```python
from build123d import *

# Parameters (mm, degrees)
F0_W      = 6
F0_H      = 10
F1_DEPTH  = 2
F2_W      = 2.8
F2_H      = 10
F3_DEPTH  = 10
F4_DEPTH  = 3
F5_DEPTH  = 0.8
F7_DEPTH  = 25
F8_SIZE   = 0.5
F10_DEPTH = 63
F11_W     = 6
F11_H     = 2
F12_DEPTH = 10
F13_W     = 2.8
F13_H     = 10
F14_DEPTH = 10
F15_R     = 2.5
F16_DEPTH = 25
F17_SIZE  = 4
F18_W     = 2.8
F18_H     = 51
F19_DEPTH = 1


with BuildPart() as f1:
    # F0 (on Top) → F1 (new body)
    with BuildSketch(Plane.XY):
        with Locations((3, -5)):
            Rectangle(F0_W, F0_H)
    extrude(amount=F1_DEPTH)

    # F2 (on face) → F3 (join)
    with BuildSketch(Plane.XY.offset(2)):
        with Locations((3, -5)):
            Rectangle(F2_W, F2_H)
    extrude(amount=F3_DEPTH)

    # F4 (cut): a face of the model
    f4_faces = [f1.faces().sort_by_distance(p)[0] for p in [
        (3, -5, 12),
    ]]
    extrude(f4_faces, amount=-F4_DEPTH, mode=Mode.SUBTRACT)

    # F5 (cut): a face of the model
    f5_faces = [f1.faces().sort_by_distance(p)[0] for p in [
        (3, 0, 3.7911392405),
    ]]
    extrude(f5_faces, amount=-F5_DEPTH, mode=Mode.SUBTRACT)

    # F6 (on face) → F7 (cut)
    with BuildSketch(Plane.YZ.offset(4.4)):
        with BuildLine():
            Line((-7.9, 9), (-7.9, 4.7))
            ThreePointArc((-7.9, 4.7), (-5.4, 2.2), (-2.9, 4.7))
            Line((-2.9, 4.7), (-2.9, 9))
            Line((-2.9, 9), (-7.9, 9))
        make_face()
    extrude(amount=-F7_DEPTH, mode=Mode.SUBTRACT)

    # F8
    f8_edges = [f1.edges().sort_by_distance(p)[0] for p in [
        (3, -7.9, 9),
        (3, -2.9, 9),
        (3, -10, 9),
        (3, -0.8, 9),
    ]]
    chamfer(f8_edges, length=F8_SIZE)

    # F9 (on face) → F10 (join)
    with BuildSketch(Plane.XZ.offset(10)):
        Polygon((1.6, 2), (0, 2), (0, 0), (6, 0), (6, 2), (4.4, 2), align=None)
    extrude(amount=F10_DEPTH)

    # F11 (on face) → F12 (join)
    with BuildSketch(Plane.XY.offset(2)):
        with Locations((3, -72)):
            Rectangle(F11_W, F11_H)
    extrude(amount=F12_DEPTH)

    # F13 (on face) → F14 (join)
    with BuildSketch(Plane(origin=(0, -71, 0), x_dir=(-1, 0, 0), z_dir=(0, 1, 0))):
        with Locations((-3, 7)):
            Rectangle(F13_W, F13_H)
    extrude(amount=F14_DEPTH)

    # F15 (on face) → F16 (cut)
    with BuildSketch(Plane(origin=(1.6, 0, 0), x_dir=(0, -1, 0), z_dir=(-1, 0, 0))):
        with Locations((68.3, 4.7)):
            Circle(F15_R)
    extrude(amount=-F16_DEPTH, mode=Mode.SUBTRACT)

    # F17
    f17_edges = [f1.edges().sort_by_distance(p)[0] for p in [
        (3, -61, 12),
    ]]
    chamfer(f17_edges, length=F17_SIZE)

    # F18 (on face) → F19 (join)
    with BuildSketch(Plane.XY.offset(2)):
        with Locations((3, -35.5)):
            Rectangle(F18_W, F18_H)
    extrude(amount=F19_DEPTH)


solid = f1.part
```
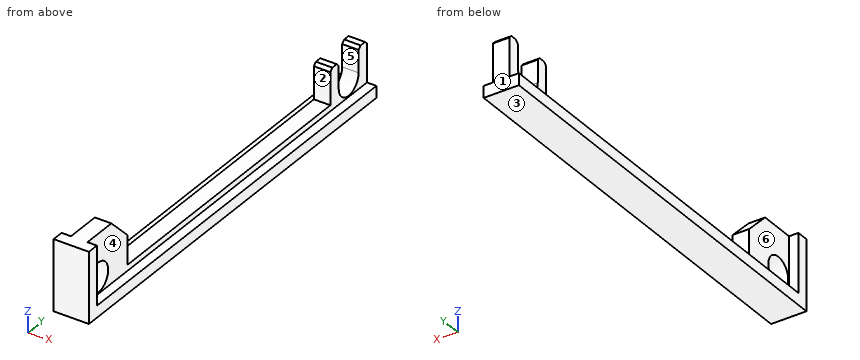
Can you work these out from the model? Positions are in its coordinate system, mm. Face numbers are marked on the shaded views. A direction names the side the tool comes from. Give positions to 0.01 mm unless a question says otherwise; leave off trailing zeros. Write each loop counter-clockwise with the first axis right and the second up, starting at its lowest first coordinate (ties: lowest second). Pieces come first, ordered by that corner, then holes. Notation, with made-up numbers: (32.5, -16.5) -> (66.5, -16.5) arc R27 cw to (66.5, 12.5) -> close; hole circle Ø4 at (-8.75, -36.75). An arc over 180 degrees is marked (long way). One line per item, written item: value.
Q1. Imagine slicing it at D-D on y = -5.4. Please give me the cut outline in (x, z).
Results found:
outline: (0, 0) -> (6, 0) -> (6, 2) -> (4.4, 2) -> (4.4, 2.2) -> (1.6, 2.2) -> (1.6, 2) -> (0, 2) -> close
Q2. Which directions (+Z, -Z, +X, -X, +Y, -Y) give clear straight access to the entire face, cutting with the end or side of a thin tool? Please do the marked faces 4, 5 and 6.
Results found:
face 4: +Z, +X, +Y
face 5: +Z, +X, -X
face 6: +Z, -X, +Y
Q3. Imagine slicing it at C-C on y = -44.5. Please give me the cut outline in (x, z).
Results found:
outline: (0, 0) -> (6, 0) -> (6, 2) -> (4.4, 2) -> (4.4, 3) -> (1.6, 3) -> (1.6, 2) -> (0, 2) -> close
Q4. For P1, Ø0.8, axis at x = 5, y = -43, coming from the +Z side; P2, Ø0.9, axis at x = 3, y = -9, coming from the +Z side; P3, Ø0.8, axis at x = 3, y = -47.5, coming from the +Z side, each with a flat end and sliding along its axis, tell me the tip position at first contact or that it passes through.
Results found:
P1: stops at z = 2
P2: stops at z = 9
P3: stops at z = 3
Q5. Imagine slicing it at B-B on x = 2.4. Please give me the cut outline in (y, z), and give its area (3 significant figures).
Results found:
outline: (-73, 0) -> (-0.8, 0) -> (-0.8, 8.5) -> (-1.3, 9) -> (-2.4, 9) -> (-2.9, 8.5) -> (-2.9, 4.7) arc R2.5 cw to (-7.9, 4.7) -> (-7.9, 8.5) -> (-8.4, 9) -> (-9.5, 9) -> (-10, 8.5) -> (-10, 3) -> (-61, 3) -> (-61, 8) -> (-65, 12) -> (-73, 12) -> close; hole circle Ø5 at (-68.3, 4.7)
area: 320 mm^2
Q6. We'd pull the mould along Y, two halves only. Please class the marked faces 1, 2 and 3: +Y half, -Y half, draft (parallel to the pull), parting line (faces both ways), or undercut.
Results found:
face 1: +Y half
face 2: undercut
face 3: draft
Q7. Imagine slicing it at A-A on y = -68.3. Please give me the cut outline in (x, z), and give its area (3 significant figures).
Results found:
outline: (0, 0) -> (6, 0) -> (6, 2) -> (4.4, 2) -> (4.4, 2.2) -> (1.6, 2.2) -> (1.6, 2) -> (0, 2) -> close; (1.6, 7.2) -> (4.4, 7.2) -> (4.4, 12) -> (1.6, 12) -> close
area: 26.0 mm^2
Q8. Please list where these lines run through material, in increasing order: line 1 (Z direction, x = 2.25, y = -68.3); line 2 (Y direction, x = 1.65, z = 4.75); line 3 (Y direction, x = 3.9, z = 7). Write a range as [from, to].
Results found:
line 1: z = [0, 2.2], [7.2, 12]
line 2: y = [-73, -70.8], [-65.8, -61], [-10, -7.9], [-2.9, -0.8]
line 3: y = [-73, -69.28], [-67.32, -61], [-10, -7.9], [-2.9, -0.8]
